Geometry: final body of the model. Coordinates: model frame, mm. Give positions to 0.01 mm unless a question says otherwise; leave off trailing zeros. Write each loop counter-clockwise with the first axis right and the second up, starting at its lowest first coordinate (ties: lowest second). Pieces come first, ordered by that corner, then holes. Notation, with made-up numbers: M -36,88.25 L 21,88.25 A13 cw 21,107.25 Z; hole C 36.5,62 d10. An arc over 180 degrees is marked long. Use one line per item in the form item = value. Start each with the question number.
Item 1: Section query A-A on x = 0. Return loops of the section in (y, z), then the cut area to 3 significant figures.
Item 2: Material intervals for line 1 along X through (y, z) = (-87, -1.7); line 2 along Y through (x, z) = (0, -0.35); line 3 along X through (y, z) = (-63.5, 2.45), sorted ascending. Write a range as from..to.
Item 3: Section query D-D on y = 104. Return loops of the section in (x, z), then the cut area to 3 significant figures.
Item 4: Pull-direction query (X, two-part tool) for faces 1 (the flat face through (85.99, -61.09, 0.04)), 2 (the flat face through (58, 2, -3)), 3 (the cylindrical face through (-107.13, -82.15, 0.04)), 4 (the flat face through (-61.09, -85.99, 0.04)); classes: released by +X, released by -X, zero draft, split by the parting line, or undercut.
Item 5: Contact query for a flat-ended pin moving along its axis: P1, Ø5, axis at x = 46.5, y = 10.5, coming from the +Z side. Output: stop coordinate, or through.
Item 6: Section query C-C on z = -1.75. Give the number of separate pieces and of enclosed holes in the cut face, then the cut area to 3 significant figures.
Autodesk Inventor part; units mm, degrees
ref_plane "YZ Plane" through (0, 0, 0) normal (1, 0, 0) x (0, 1, 0)
ref_plane "XZ Plane" through (0, 0, 0) normal (0, 1, 0) x (-1, 0, 0)
ref_plane "XY Plane" through (0, 0, 0) normal (0, 0, 1) x (1, 0, 0)
sketch "Эскиз1" plane through (0, 0, 0) normal (0, 0, 1) x (1, 0, 0)
  circle A0 centre (0, 0) radius 135
  dimension "d0" = 270
extrude "Выдавливание1" add sketch "Эскиз1" along normal mid plane 6
sketch "Эскиз3" plane through (0, 0, -3) normal (0, 0, -1) x (-1, 0, 0)
  circle A0 centre (0, 0) radius 50
  dimension "d14" = 100
extrude "Выдавливание2" cut sketch "Эскиз3" against normal through all
sketch "Эскиз4" plane through (0, 0, 3) normal (0, 0, 1) x (1, 0, 0)
  circle A0 centre (0, 0) radius 101 construction
  circle A1 centre (0, 101) radius 26.5 construction
  line L0 (0, 0) -> (118.5479, 118.5479) construction
  line L1 (0, 0) -> (0, 152.163) construction
  line L2 (86.9741, 51.6188) -> (51.6188, 86.9741)
  line L3 (51.6188, 86.9741) -> (55.8614, 91.2168)
  line L4 (55.8614, 91.2168) -> (91.2168, 55.8614)
  line L5 (91.2168, 55.8614) -> (86.9741, 51.6188)
  line L6 (86.9741, 51.6188) -> (55.8614, 91.2168) construction
  line L7 (51.6188, 86.9741) -> (91.2168, 55.8614) construction
  line L8 (66.468, 80.6102) -> (62.2254, 76.3675)
  line L9 (80.6102, 66.468) -> (76.3675, 62.2254)
  point P0 (71.4178, 71.4178)
  dimension "d17" = 202
  dimension "d18" = 53
  dimension "d19" = 45
  dimension "d20" = 6
  dimension "d21" = 50
  dimension "d22" = 15
extrude "Выдавливание3" cut sketch "Эскиз4" against normal through all contours L2 L9 L4 L5 | L2 L3 L4 L8
pattern_circular "Круговой массив2" count 4 over 360 about axis through (0, 0, 0) along (0, 0, 1) of "Выдавливание3"
properties part number "Диск_опорный_В5" material "По умолчанию1"
Answer sheet:
q1.outline = M -135,-3 L -50,-3 L -50,3 L -135,3 Z; M 50,-3 L 135,-3 L 135,3 L 50,3 Z
q1.area = 1,020 mm2
q2.line_1 = -103.23..-60.08, -51.64..51.64, 60.08..103.23
q2.line_2 = -135..-50, 50..135
q2.line_3 = -119.13..-83.58, -77.64..77.64, 83.58..119.13
q3.outline = M -86.08,-3 L 86.08,-3 L 86.08,3 L -86.08,3 Z
q3.area = 1,030 mm2
q4.face_1 = undercut
q4.face_2 = zero draft
q4.face_3 = split by the parting line
q4.face_4 = undercut
q5.P1 = 3
q6.separate_pieces = 1
q6.enclosed_holes = 9
q6.area = 48,700 mm2
